Answer from the drawing. Dimensions are ordinates in mm from the lowest x, y and z of the part. A direction names the side the tool comes from. Give positions to 0.01 mm unless a question says otherwise; leave off trailing zeros. Loops run counter-clockwise (first coordinate to the right, second up) from the corner with the lowest first, then second, coordinate; pieces in that order, holes last.
Item 1: A tool of negligible diameter and unlimited length cuts with its end or side. For the marked faces 4 and 5, from which of +Z, -Z, +X, -X, +Y, -Y can it reach the whole face along a straight path? Write none if from no direction.
Item 2: Consider line 1 along X through (y, z) = (15.25, 60); line 2 along Z through (x, y) = (12, 11.5); line 3 along Y through (x, z) = (58, 43). Determine where each line is inside the solid, lowest interval first.
Item 3: Section A-A, the plane x = 10.5 is taken. Give the vertices of the cut face in (y, z), and give its area (4 significant figures).
Item 4: Each of these flat-tipped pins is pushed along its axis until it touches: pin 1 Ø2 at (x, z) = (50.5, 18) entering from -Y; pin 2 Ø0.8 at (y, z) = (8.5, 1) entering from +X; pin 3 Ø8 at (y, z) = (4, 57.5) entering from -X; pin 4 Ø9 at (x, y) = (40.5, 8.5) entering from -Z. Where does it stop, or does it pass through?
Item 5: Section D-D, the plane y = 3.75 is taken. Give the vertices of the cut face in (x, z).
Item 6: The mould has two halves that part along X. Classify the marked faces 1, 2 and 3: pulls with the +X half, pulls with the -X half, needs draft (parallel to the pull), parting line crosses it, or undercut.
Item 7: Section B-B, the plane y = 16.5 is taken. Give the vertices of the cut face in (x, z).
Item 8: Section C-C, the plane z = 47 is taken. Give the vertices of the cut face in (x, y), and give its area (4 significant figures).
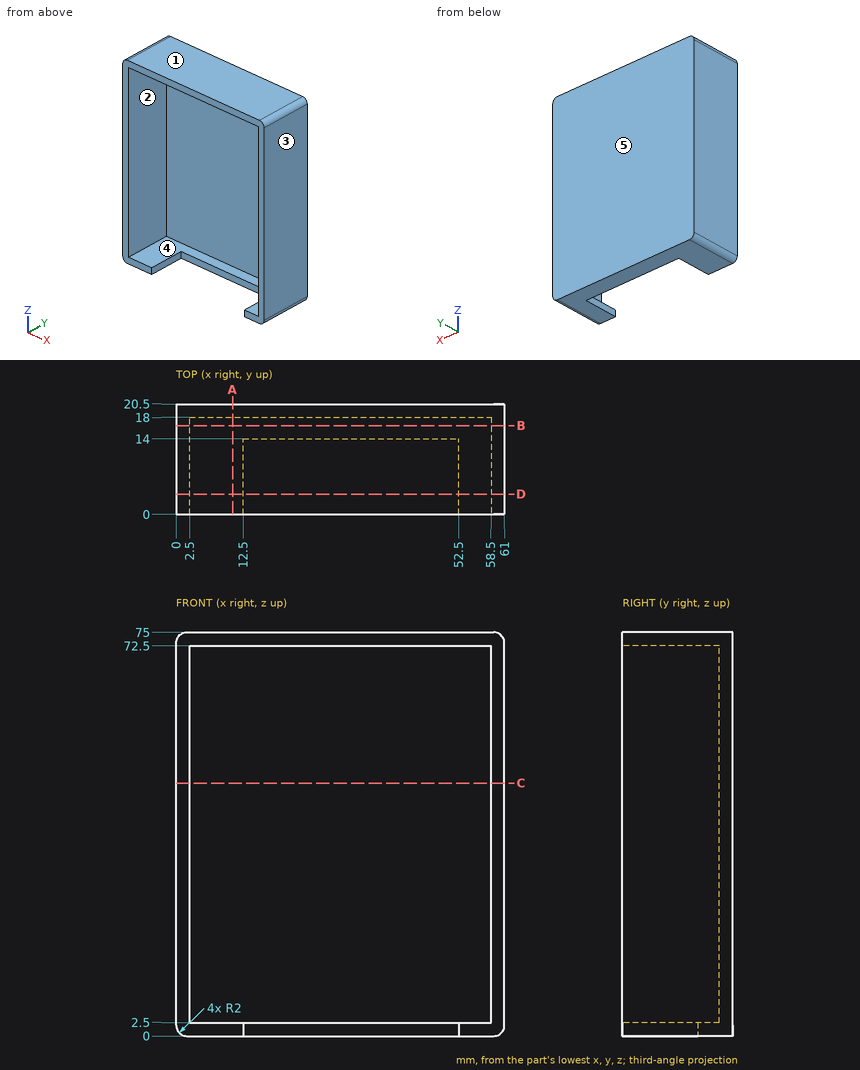
Worked answers:
1. face 4: -Y
1. face 5: +Z, -Z, +X, -X, +Y
2. line 1: x = 0 to 2.5, 58.5 to 61
2. line 2: z = 0 to 2.5, 72.5 to 75
2. line 3: y = 18 to 20.5
3. outline: (0, 0) - (20.5, 0) - (20.5, 75) - (0, 75) - (0, 72.5) - (18, 72.5) - (18, 2.5) - (0, 2.5) - close
3. area: 277.5 mm2
4. pin 1: stops at y = 18
4. pin 2: stops at x = 60.91
4. pin 3: stops at x = 0
4. pin 4: stops at z = 72.5
5. outline: (0, 2) arc R2 ccw to (2, 0) - (12.5, 0) - (12.5, 2.5) - (2.5, 2.5) - (2.5, 72.5) - (58.5, 72.5) - (58.5, 2.5) - (52.5, 2.5) - (52.5, 0) - (59, 0) arc R2 ccw to (61, 2) - (61, 73) arc R2 ccw to (59, 75) - (2, 75) arc R2 ccw to (0, 73) - close
6. face 1: needs draft
6. face 2: undercut
6. face 3: pulls with the +X half
7. outline: (0, 2) arc R2 ccw to (2, 0) - (59, 0) arc R2 ccw to (61, 2) - (61, 73) arc R2 ccw to (59, 75) - (2, 75) arc R2 ccw to (0, 73) - close; hole (2.5, 2.5) - (58.5, 2.5) - (58.5, 72.5) - (2.5, 72.5) - close
8. outline: (0, 0) - (2.5, 0) - (2.5, 18) - (58.5, 18) - (58.5, 0) - (61, 0) - (61, 20.5) - (0, 20.5) - close
8. area: 242.5 mm2
